```python
from build123d import *

# Parameters (mm, degrees)
F1_DEPTH      = 6.35
F1_DEPTH_BACK = 6.35
F3_D          = 4.0386
F4_R          = 1.27


with BuildPart() as f1:
    # F0 (on Front) → F1 (new body, two sides)
    with BuildSketch(Plane.XZ) as f1_sk:
        Polygon((-6.35, 19.05), (6.35, 19.05), (6.35, -19.05), (-6.35, -19.05), (-6.35, -15.875), (-9.525, -15.875), (-9.525, -22.225), (9.525, -22.225), (9.525, 22.225), (-9.525, 22.225), (-9.525, 15.875), (-6.35, 15.875), align=None)
    extrude(amount=F1_DEPTH)
    extrude(f1_sk.sketch, amount=-F1_DEPTH_BACK)

    # F3 (through all)
    with Locations(Plane.XY.offset(22.225)):
        with Locations((0, 0)):
            Hole(F3_D / 2)

    # F4
    f4_edges = [f1.edges().sort_by_distance(p)[0] for p in [
        (-9.525, 0, 22.225),
        (-9.525, 0, 15.875),
        (-6.35, 0, 15.875),
        (9.525, 0, 22.225),
        (9.525, 0, -22.225),
        (-9.525, 0, -22.225),
        (-9.525, 0, -15.875),
        (-6.35, 0, -15.875),
    ]]
    fillet(f4_edges, radius=F4_R)


solid = f1.part
```
Here's how the part is built. I have some questions about the finished solid (model axes, mm). A direction names the side the tool comes from. Coordinates: 2 decimals unless noted, no trailing zeros. Order: outer loops, then holes, each group sorted by start corner. A loop starts at its lowest first (then second) coordinate and runs counter-clockwise, first axis right, second up. Notation, with made-up numbers: (-23, -21) -> (-16, -21) arc R20 ccw to (-16, 7) -> close; hole circle Ø6 at (-9.5, 10.25). An arc over 180 degrees is marked (long way). Return JSON: item names as keys, results as strings.
1) Thinking about a two-plate mould opening in Z: for faces 4 (the cylindrical face through (-6.71, 0.09, 16.26)), 5 (the flat face through (-9.525, 0, 19)), 6 (the cylindrical face through (-9.143, -0.089, 21.863)), which applies, +Z half, -Z half, draft (parallel to the pull), parting line (faces both ways), or undercut?
Conclusion:
{"face 4": "undercut", "face 5": "draft", "face 6": "+Z half"}
2) If we section it at C-C on z = -4: List the corners of the cut face in (x, y) for me (3 decimals), plus the area to 3 significant figures.
Conclusion:
{"outline": "(6.35, -6.35) -> (9.525, -6.35) -> (9.525, 6.35) -> (6.35, 6.35) -> close", "area": "40.3 mm²"}
3) If we section it at D-D on y = 3: List the corners of the cut face in (x, z) for me (3 decimals), plus the area to 3 significant figures.
Conclusion:
{"outline": "(-9.525, -20.955) arc R1.27 ccw to (-8.255, -22.225) -> (8.255, -22.225) arc R1.27 ccw to (9.525, -20.955) -> (9.525, 20.955) arc R1.27 ccw to (8.255, 22.225) -> (-8.255, 22.225) arc R1.27 ccw to (-9.525, 20.955) -> (-9.525, 17.145) arc R1.27 ccw to (-8.255, 15.875) -> (-7.62, 15.875) arc R1.27 ccw to (-6.35, 17.145) -> (-6.35, 19.05) -> (6.35, 19.05) -> (6.35, -19.05) -> (-6.35, -19.05) -> (-6.35, -17.145) arc R1.27 ccw to (-7.62, -15.875) -> (-8.255, -15.875) arc R1.27 ccw to (-9.525, -17.145) -> close", "area": "259 mm²"}
4) I'm going to push flat-ended pins straight in: P1, Ø4.5, axis at x = 0, y = 0, coming from the +Z side (3 decimals); P2, Ø4, axis at y = -2, z = 9, coming from the -X side. Where does each tip first touch, or does it pass through?
Conclusion:
{"P1": "stops at z = 22.225", "P2": "stops at x = 6.35"}
5) On a 3-axis mill with a long thin cutter (end or side, diameter ignored), from which of +Z, -Z, +X, -X, +Y, -Y can I reach the whole of each face in a straight line? I mean faces 1 (the flat face through (-9.525, 0, -19)), 2 (the cylindrical face through (-6.71, -0.09, -16.26)), 3 (the cylindrical face through (-9.143, -0.089, -16.237)). Say none if no direction works.
Conclusion:
{"face 1": "+Z, -Z, -X, +Y, -Y", "face 2": "+Y, -Y", "face 3": "-X, +Y, -Y"}
6) If we section it at B-B on y = 0: List the corners of the cut face in (x, z) for me (3 decimals).
Conclusion:
{"outline": "(-9.525, -20.955) arc R1.27 ccw to (-8.255, -22.225) -> (-2.019, -22.225) -> (-2.019, -19.05) -> (-6.35, -19.05) -> (-6.35, -17.145) arc R1.27 ccw to (-7.62, -15.875) -> (-8.255, -15.875) arc R1.27 ccw to (-9.525, -17.145) -> close; (-9.525, 17.145) arc R1.27 ccw to (-8.255, 15.875) -> (-7.62, 15.875) arc R1.27 ccw to (-6.35, 17.145) -> (-6.35, 19.05) -> (-2.019, 19.05) -> (-2.019, 22.225) -> (-8.255, 22.225) arc R1.27 ccw to (-9.525, 20.955) -> close; (2.019, -22.225) -> (8.255, -22.225) arc R1.27 ccw to (9.525, -20.955) -> (9.525, 20.955) arc R1.27 ccw to (8.255, 22.225) -> (2.019, 22.225) -> (2.019, 19.05) -> (6.35, 19.05) -> (6.35, -19.05) -> (2.019, -19.05) -> close"}
7) If I drill on probe 1 along Z at (x, y) = (0, 2.75) (3 decimals); probe 2 along Y at (x, z) = (0, -19.7); probe 3 along X at (y, z) = (5.5, 19) (3 decimals), over which ranges is the centre line in solid material (lowest first)?
Conclusion:
{"probe 1": "z = -22.225 to -19.05, 19.05 to 22.225", "probe 2": "y = -6.35 to -2.02, 2.02 to 6.35", "probe 3": "x = -9.525 to -6.35, 6.35 to 9.525"}
8) If we section it at A-A on x = 0: List the corners of the cut face in (y, z) for me (3 decimals), plus the area to 3 significant figures.
Conclusion:
{"outline": "(-6.35, -22.225) -> (-2.019, -22.225) -> (-2.019, -19.05) -> (-6.35, -19.05) -> close; (-6.35, 19.05) -> (-2.019, 19.05) -> (-2.019, 22.225) -> (-6.35, 22.225) -> close; (2.019, -22.225) -> (6.35, -22.225) -> (6.35, -19.05) -> (2.019, -19.05) -> close; (2.019, 19.05) -> (6.35, 19.05) -> (6.35, 22.225) -> (2.019, 22.225) -> close", "area": "55.0 mm²"}
